Geometry check sheet. Reference: the model listing, model coordinates, mm. Coordinates: 2 decimals unless noted, no trailing zeros. Order: outer loops, then holes, each group sorted by start corner. A loop starts at its lowest first (then second) coordinate and runs counter-clockwise, first axis right, second up.
```python
from build123d import *

# Parameters (mm, degrees)
F0_W     = 50.8
F0_H     = 914.4
F1_DEPTH = 50.8
F2_T     = -2.54


with BuildPart() as f1:
    # F0 (on Front) → F1 (new body)
    with BuildSketch(Plane.XZ):
        with Locations((25.4, 457.2)):
            Rectangle(F0_W, F0_H)
        Polygon((50.8, 0), (0, 0), (-355.6, 0), (-355.6, -50.8), (406.4, -50.8), (406.4, 0), align=None)
    extrude(amount=F1_DEPTH)

    # F2
    f2_openings = [f1.faces().sort_by_distance(p)[0] for p in [
        (25.4, -25.4, 914.4),
        (406.4, -25.4, -25.4),
        (-355.6, -25.4, -25.4),
    ]]
    offset(amount=F2_T, openings=f2_openings, kind=Kind.INTERSECTION)


solid = f1.part
```
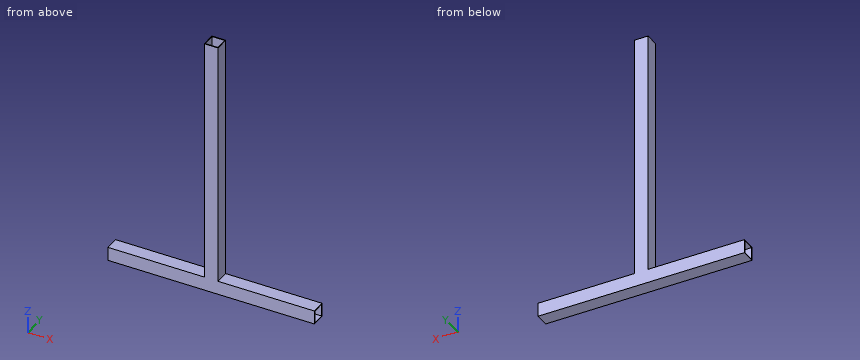
Item 1: Sectioned sample at B-B (x = -15). Record the cut outline in (y, z).
Item 2: Depth check by flat-ended pin: P1, Ø1.5, axis at y = -44.5, z = 451.5, coming from the -X side; P2, Ø3, axis at y = -10.5, z = 698, coming from the +X side. Enter the tip coordinate at first touch or a pass-through.
Item 3: Thickness scan on line 1 along Z through (x, y) = (282, -47); line 2 along X through (y, z) = (-22.5, 694.5). Record the ranges inside material, lowest first.
Item 4: Sectioned sample at A-A (y = -19). Record the cut outline in (x, z), and give its area (3 significant figures).
Item 5: Sectioned sample at C-C (z = 95). Record the cut outline in (x, y), and give its area (3 significant figures).
Geometry check:
1. outline: (-50.8, -50.8) - (0, -50.8) - (0, 0) - (-50.8, 0) - close; hole (-48.26, -48.26) - (-2.54, -48.26) - (-2.54, -2.54) - (-48.26, -2.54) - close
2. P1: stops at x = 0
2. P2: stops at x = 50.8
3. line 1: z = -50.8 to -48.26, -2.54 to 0
3. line 2: x = 0 to 2.54, 48.26 to 50.8
4. outline: (-355.6, -50.8) - (406.4, -50.8) - (406.4, -48.26) - (-355.6, -48.26) - close; (-355.6, -2.54) - (2.54, -2.54) - (2.54, 914.4) - (0, 914.4) - (0, 0) - (-355.6, 0) - close; (48.26, -2.54) - (406.4, -2.54) - (406.4, 0) - (50.8, 0) - (50.8, 914.4) - (48.26, 914.4) - close
4. area: 8,400 mm2
5. outline: (0, -50.8) - (50.8, -50.8) - (50.8, 0) - (0, 0) - close; hole (2.54, -48.26) - (48.26, -48.26) - (48.26, -2.54) - (2.54, -2.54) - close
5. area: 490 mm2
